from build123d import *

# Parameters (mm, degrees)
SKETCH1_W           = 35
SKETCH1_H           = 60
BOSS_EXTRUDE1_DEPTH = 4


with BuildPart() as part:
    # Sketch1 → Boss-Extrude1 (new, symmetric)
    with BuildSketch(Plane.XY):
        Rectangle(SKETCH1_W, SKETCH1_H)
    extrude(amount=BOSS_EXTRUDE1_DEPTH, both=True)

    # Sketch3 → M6 Clearance Hole1 (revolve, cut)
    with BuildSketch(Plane(origin=(-12.5, 25, 4), x_dir=(0, -1, 0), z_dir=(1, 0, 0))):
        Polygon((0, 0), (0, 9.982840043), (3.3, 8), (3.3, 0), align=None)
    m6_clearance_hole1 = revolve(axis=Axis((-12.5, 25, 10.35), (0, 0, -1)), mode=Mode.SUBTRACT)

    # Mirror1: M6 Clearance Hole1 across plane
    add(m6_clearance_hole1.mirror(Plane(origin=(0, 0, 0), x_dir=(0, 0, 1), z_dir=(1, 0, 0))), mode=Mode.SUBTRACT)

    # Mirror2: M6 Clearance Hole1 across plane
    add(m6_clearance_hole1.mirror(Plane.ZX), mode=Mode.SUBTRACT)

    # Mirror2 copy 1 sketch → Mirror2 copy 1 (revolve, cut)
    with BuildSketch(Plane(origin=(12.5, -25, 4), x_dir=(0, 1, 0), z_dir=(-1, 0, 0))):
        Polygon((0, 0), (0, 9.982840043), (3.3, 8), (3.3, 0), align=None)
    revolve(axis=Axis((12.5, -25, 10.35), (0, 0, -1)), mode=Mode.SUBTRACT)


solid = part.part
Source: CAD feature listing. Evaluate the final solid. Frame: model axes, mm. Round coordinates to 2 decimals unless told otherwise and drop trailing zeros. Order: outer loops, then holes, each group sorted by start corner. A loop starts at its lowest first (then second) coordinate and runs counter-clockwise, first axis right, second up. Notation, with made-up numbers: (69.5, 54.25) - (118.5, 54.25) arc R21 ccw to (118.5, 68.25) - close; hole circle Ø6 at (40, -5.75). An arc over 180 degrees is marked (long way). Use a Markdown table: item, result. Add a question column.
1. Section query A-A (x = 12.5). Return the cut outline in (y, z).
2. Line query: probe 1 along Y at (x, z) = (-12.5, -2); probe 2 along X at (y, z) = (-25, -2); probe 3 along X at (y, z) = (24, 3.5). Output: solid intervals per line, ascending.
3. Mould query, pull axis Y, two halves, no side actions, for faces 1 (the flat face through (0, -30, 0)), 2 (the cylindrical face through (-11.24, -21.95, 0.06)), 3 (the flat face through (0, 0, -4)), 4 (the cylindrical face through (-11.24, 21.95, 0.06)). Classes: +Y half, -Y half, draft (parallel to the pull), parting line (faces both ways), or undercut.
4. Section query C-C (y = -25). Return the cut outline in (x, z).
5. Section query B-B (z = 0.5). Return the cut outline in (x, y).
Derived:
| question | item | result |
|---|---|---|
| 1 | outline | (-30, -4) - (-28.3, -4) - (-28.3, 4) - (-30, 4) - close; (-21.7, -4) - (21.7, -4) - (21.7, 4) - (-21.7, 4) - close; (28.3, -4) - (30, -4) - (30, 4) - (28.3, 4) - close |
| 2 | probe 1 | -30 to -28.3, -21.7 to 21.7, 28.3 to 30 |
| 2 | probe 2 | -17.5 to -15.8, -9.2 to 9.2, 15.8 to 17.5 |
| 2 | probe 3 | -17.5 to -15.64, -9.36 to 9.36, 15.64 to 17.5 |
| 3 | face 1 | -Y half |
| 3 | face 2 | undercut |
| 3 | face 3 | draft |
| 3 | face 4 | undercut |
| 4 | outline | (-17.5, -4) - (-15.8, -4) - (-15.8, 4) - (-17.5, 4) - close; (-9.2, -4) - (9.2, -4) - (9.2, 4) - (-9.2, 4) - close; (15.8, -4) - (17.5, -4) - (17.5, 4) - (15.8, 4) - close |
| 5 | outline | (-17.5, -30) - (17.5, -30) - (17.5, 30) - (-17.5, 30) - close; hole circle Ø6.6 at (-12.5, -25); hole circle Ø6.6 at (-12.5, 25); hole circle Ø6.6 at (12.5, -25); hole circle Ø6.6 at (12.5, 25) |
